Source: CAD feature listing. Evaluate the final solid. Frame: model axes, mm. A direction names the side the tool comes from. Give positions to 0.01 mm unless a question says otherwise; leave off trailing zeros. Order: outer loops, then holes, each group sorted by start corner. A loop starts at its lowest first (then second) coordinate and runs counter-clockwise, first axis right, second up.
1) Section B-B, the plane z = 143. Return loops of the section in (x, y), plus the area to 3 significant figures.
2) Section C-C, the plane y = -1.5. Return loops of the section in (x, z), plus the area to 3 significant figures.
3) Section A-A, the plane x = 0. Return loops of the section in (y, z) (3 decimals).
4) Draft query along Z for faces 3 (the face through (0, 0, 0)), 4 (the face through (0, -1, 215.9)), 5 (the face through (-0.867, -3.905, 106.439)), 6 (the face through (0, 2.54, 57)). Return one class per face: released by +Z, released by -Z, zero draft, split by the parting line, or undercut.
5) Section D-D, the plane z = 22.5. Return loops of the section in (x, y), plus the area to 3 significant figures.
6) First-contact query: P1, Ø2, axis at y = -1, z = 118.5, coming from the +X side; P2, Ø2, axis at x = -2, z = 71.5, coming from the -Y side; P3, Ø1.6, axis at x = 0, y = 3.5, coming from the +Z side (3 decimals); P4, Ø2, axis at x = -2.5, z = 73, coming from the +Y side. Flat tips, straight axial feed; report the tip coordinate or a pass-through.
7) Material intervals for line 1 (Z direction, x = 1.5, y = 3) (3 decimals); line 2 (X direction, y = 0.25, z = 143.5); line 3 (X direction, y = -2.5, z = 147.5), sorted ascending.
8) Access query for faces 1 (the face through (0, 2.54, 20)), 2 (the face through (0, 2.54, 208)). Directions: +Z, -Z, +X, -X, +Y, -Y. A direction counts if a zero-diameter tool reaches every point of the face in a straight line with its end or side. Return the directions, or none.
```python
from build123d import *

# Parameters (mm, degrees)
SKETCH1_R           = 4
BOSS_EXTRUDE1_DEPTH = 215.9
SKETCH2_W           = 12.7
SKETCH2_H           = 1.46
SKETCH2_W_2         = 25.4
SKETCH2_W_3         = 15.875
SKETCH2_W_4         = 11.43
CUT_EXTRUDE1_DEPTH  = 6.35


with BuildPart() as part:
    # Sketch1 → Boss-Extrude1 (new body)
    with BuildSketch(Plane.XY):
        Circle(SKETCH1_R)
    extrude(amount=BOSS_EXTRUDE1_DEPTH)

    # Sketch2 → Cut-Extrude1 (cut, symmetric)
    with BuildSketch(Plane(origin=(0, 0, 0), x_dir=(0, 0, -1), z_dir=(1, 0, 0))):
        with Locations((-57.15, 3.27)):
            Rectangle(SKETCH2_W, SKETCH2_H)
        with Locations((-161.925, 3.27)):
            Rectangle(SKETCH2_W_2, SKETCH2_H)
        with Locations((-207.9625, 3.27)):
            Rectangle(SKETCH2_W_3, SKETCH2_H)
        with Locations((-19.685, 3.27)):
            Rectangle(SKETCH2_W_4, SKETCH2_H)
    extrude(amount=CUT_EXTRUDE1_DEPTH, both=True, mode=Mode.SUBTRACT)


solid = part.part
```
From the geometry:
1. outline: circle Ø8 at (0, 0)
1. area: 50.3 mm2
2. outline: (-3.71, 0) - (3.71, 0) - (3.71, 215.9) - (-3.71, 215.9) - close
2. area: 1,600 mm2
3. outline: (-4, 0) - (4, 0) - (4, 13.97) - (2.54, 13.97) - (2.54, 25.4) - (4, 25.4) - (4, 50.8) - (2.54, 50.8) - (2.54, 63.5) - (4, 63.5) - (4, 149.225) - (2.54, 149.225) - (2.54, 174.625) - (4, 174.625) - (4, 200.025) - (2.54, 200.025) - (2.54, 215.9) - (-4, 215.9) - close
4. face 3: released by -Z
4. face 4: released by +Z
4. face 5: zero draft
4. face 6: undercut
5. outline: (-3.09, 2.54) arc R4 ccw (long way) to (3.09, 2.54) - close
5. area: 44.0 mm2
6. P1: stops at x = 4
6. P2: stops at y = -3.87
6. P3: stops at z = 200.025
6. P4: stops at y = 3.71
7. line 1: z = 0 to 13.97, 25.4 to 50.8, 63.5 to 149.225, 174.625 to 200.025
7. line 2: x = -3.99 to 3.99
7. line 3: x = -3.12 to 3.12
8. face 1: +X, -X, +Y
8. face 2: +Z, +X, -X, +Y
